```python
from build123d import *

# Parameters (mm, degrees)
SKETCH055_R       = 2.25
PAD023_DEPTH      = 10
SKETCH056_W       = 4.7
SKETCH056_H       = 4
PAD024_DEPTH      = 31
SKETCH057_W       = 9.7
SKETCH057_H       = 4.7
PAD025_DEPTH      = 5
SKETCH058_W       = 14.85
SKETCH058_H       = 7.35
POCKET028_DEPTH   = 7
POCKET028_FACE1_W = 3
POCKET028_FACE1_H = 14.85
POCKET029_DEPTH   = 1
POCKET029_FACE4_W = 3
POCKET029_FACE4_H = 14.85
POCKET030_DEPTH   = 1
FILLET005_R       = 12
CHAMFER002_SIZE2  = 10
CHAMFER002_SIZE   = 1.7


with BuildPart() as part:
    # Sketch055 → Pad023 (new body)
    with BuildSketch(Plane.XZ):
        Polygon((-10.15, 29.65), (-10.15, -10.65), (0, -10.65), (0, -18), (-14.85, -18), (-14.85, 37), (0, 37), (0, 29.65), align=None)
        with Locations((-6, 34.45)):
            Circle(SKETCH055_R, mode=Mode.SUBTRACT)
        with Locations((-6, -15.5)):
            Circle(SKETCH055_R, mode=Mode.SUBTRACT)
    extrude(amount=-PAD023_DEPTH)

    # Sketch056 (on Face8 of Pad023) → Pad024 (join)
    with BuildSketch(Plane(origin=(-14.85, 0, 0), x_dir=(0, 0, -1), z_dir=(-1, 0, 0))):
        with Locations((6.5, -2)):
            Rectangle(SKETCH056_W, SKETCH056_H)
    extrude(amount=PAD024_DEPTH)

    # Sketch057 (on Face7 of Pad024) → Pad025 (join)
    with BuildSketch(Plane(origin=(0, 4, 0), x_dir=(1, 0, 0), z_dir=(0, 1, 0))):
        with Locations((-41, 6.5)):
            Rectangle(SKETCH057_W, SKETCH057_H)
    extrude(amount=PAD025_DEPTH)

    # Sketch058 (on Face5 of Pad025) → Pocket028 (cut)
    with BuildSketch(Plane(origin=(0, 10, 0), x_dir=(1, 0, 0), z_dir=(0, 1, 0))):
        with Locations((-7.425, 14.325)):
            Rectangle(SKETCH058_W, SKETCH058_H)
        with Locations((-7.425, -33.325)):
            Rectangle(SKETCH058_W, SKETCH058_H)
    extrude(amount=-POCKET028_DEPTH, mode=Mode.SUBTRACT)

    # Pocket028 Face1 → Pocket029 (cut)
    with BuildSketch(Plane(origin=(-7.425, 1.5, 37), x_dir=(0, 1, 0), z_dir=(0, 0, 1))):
        Rectangle(POCKET028_FACE1_W, POCKET028_FACE1_H)
    extrude(amount=-POCKET029_DEPTH, mode=Mode.SUBTRACT)

    # Pocket029 Face4 → Pocket030 (cut)
    with BuildSketch(Plane(origin=(-7.425, 1.5, -18), x_dir=(0, -1, 0), z_dir=(0, 0, -1))):
        Rectangle(POCKET029_FACE4_W, POCKET029_FACE4_H)
    extrude(amount=-POCKET030_DEPTH, mode=Mode.SUBTRACT)

    # Fillet005
    fillet005_edges = [part.edges().sort_by_distance(p)[0] for p in [
        (-14.85, 2, -4.15),
    ]]
    fillet(fillet005_edges, radius=FILLET005_R)

    # Chamfer002
    chamfer002_edges = [part.edges().sort_by_distance(p)[0] for p in [
        (-14.85, 2, -8.85),
    ]]
    chamfer002_side = part.faces().sort_by_distance((-14.85, 5.179134, 11.284665))[0]
    chamfer(chamfer002_edges, length=CHAMFER002_SIZE, length2=CHAMFER002_SIZE2, reference=chamfer002_side)

    # Mirrored002: part across YZ


with BuildPart() as part_1:
    add(part.part)
    add(part.part.mirror(Plane.YZ))


with BuildPart() as part_2:
    # Body012 placement: moved
    add(part_1.part.moved(Location((0, 13.9, 0))))


solid = part_2.part
```
Model file for the job. Use its own axes, mm. A direction names the side the tool comes from. Give positions to 0.01 mm unless a question says otherwise; leave off trailing zeros. Write each loop counter-clockwise with the first axis right and the second up, starting at its lowest first coordinate (ties: lowest second). Pieces come first, ordered by that corner, then holes. Notation, with made-up numbers: (41, -36) - (63, -36) arc R30 ccw to (63, 3) - close; hole circle Ø2 at (56, 81). An arc over 180 degrees is marked (long way). One line per question, with ' | ' between items. Start each with the question number.
(1) Slice it at C-C on y = 21.25. Write the cut outline in (x, z).
(2) Slice it at B-B on z = -7.5. Write the cut outline in (x, y).
(3) Pin check, flat tips, straight feed: P1, Ø1.4, axis at x = 41.5, z = -6.5, coming from the +Y side; P2, Ø4, axis at x = -25, y = 19, coming from the +Z side; P3, Ø5, axis at x = 4, z = -13, coming from the +Y side. Stop position of each tip, or through.
(4) Slice it at A-A on x = -6. Write the cut outline in (y, z).
(5) Two-plate mould, pull along Z, no slides. Class faces 1 (the face through (6.07, 15.38, 32.2)), 2 (the face through (41, 22.9, -7)), 3 (the face through (-13, 20, -10.65)): +Z half, -Z half, draft (parallel to the pull), parting line (faces both ways), or undercut.
(6) 3-axis set-ups, long thin cutter, end or side, ignore diameter. For faces 4 (the face through (36.15, 20, -6)), 5 (the face through (0, 15, 29.65)), 6 (the face through (0, 16.9, 33)): which of +Z, -Z, +X, -X, +Y, -Y reach the whole face in a straight line?
(7) Wall check: line 1 along X through (y, z) = (15.05, -15.5); line 2 along X through (y, z) = (19, -4.5); line 3 along X through (y, z) = (16, 21). Give the ranges that are in metal, low to high. Write a range as from..to.
(8) Slice it at D-D on z = 34.45. Write the cut outline in (x, y), plus the area to 3 significant figures.
Results below:
1) outline: (-45.85, -8.85) - (-36.15, -8.85) - (-36.15, -4.15) - (-45.85, -4.15) - close; (-14.85, -10.65) - (-10.15, -10.65) - (-10.15, 29.65) - (-14.85, 29.65) - close; (10.15, -10.65) - (14.85, -10.65) - (14.85, 29.65) - (10.15, 29.65) - close; (36.15, -8.85) - (45.85, -8.85) - (45.85, -4.15) - (36.15, -4.15) - close
2) outline: (-45.85, 13.9) - (-10.15, 13.9) - (-10.15, 23.9) - (-14.85, 23.9) - (-14.85, 17.9) - (-36.15, 17.9) - (-36.15, 22.9) - (-45.85, 22.9) - close; (10.15, 13.9) - (45.85, 13.9) - (45.85, 22.9) - (36.15, 22.9) - (36.15, 17.9) - (14.85, 17.9) - (14.85, 23.9) - (10.15, 23.9) - close
3) P1: y = 22.9 | P2: z = -3.62 | P3: y = 16.9
4) outline: (13.9, -13.25) - (16.9, -13.25) - (16.9, -10.65) - (13.9, -10.65) - close; (13.9, 29.65) - (16.9, 29.65) - (16.9, 32.2) - (13.9, 32.2) - close
5) face 1: undercut | face 2: draft | face 3: -Z half
6) face 4: +Z, -Z, +Y | face 5: +Y, -Y | face 6: +Z, +X, -X, +Y
7) line 1: -14.85..-8.25, -3.75..3.75, 8.25..14.85 | line 2: -45.85..-36.15, -14.85..-10.15, 10.15..14.85, 36.15..45.85 | line 3: -14.85..-10.15, 10.15..14.85
8) outline: (-14.85, 13.9) - (-8.25, 13.9) - (-8.25, 16.9) - (-14.85, 16.9) - close; (-3.75, 13.9) - (3.75, 13.9) - (3.75, 16.9) - (-3.75, 16.9) - close; (8.25, 13.9) - (14.85, 13.9) - (14.85, 16.9) - (8.25, 16.9) - close | area: 62.1 mm^2
